```python
from build123d import *

# Parameters (mm, degrees)
F0_W     = 50.8
F0_H     = 50.8
F1_DEPTH = 387.35
F2_SIZE  = 50.79999
F3_W     = 44.45
F3_H     = 44.45
F4_DEPTH = 876.3
F5_R     = 9.525
F7_D     = 12.7
F7_DEPTH = 127
F7_TIP   = 3.8154649308


# Not quite as in the source:
# - a fillet or chamfer is up to 0.001 mm smaller than in the source, because OpenCascade refuses the exact size


with BuildPart() as f1:
    # F0 (on Right) → F1 (new body)
    with BuildSketch(Plane.YZ):
        with Locations((25.4, 25.4)):
            Rectangle(F0_W, F0_H)
    extrude(amount=-F1_DEPTH)

    # F2 (size 50.8 in the source; OpenCascade refuses exactly that, so slightly less here)
    f2_edges = [f1.edges().sort_by_distance(p)[0] for p in [
        (-387.35, 50.8, 25.4),
    ]]
    chamfer(f2_edges, length=F2_SIZE)

    # F3 (on face) → F4 (cut)
    with BuildSketch(Plane.YZ):
        with Locations((25.4, 25.4)):
            Rectangle(F3_W, F3_H)
    extrude(amount=-F4_DEPTH, mode=Mode.SUBTRACT)

    # F5
    f5_edges = [f1.edges().sort_by_distance(p)[0] for p in [
        (-192.087505, 3.175, 3.175),
        (-169.862505, 47.625, 3.175),
        (-169.862505, 47.625, 47.625),
        (-192.087505, 3.175, 47.625),
        (-168.275005, 50.8, 0),
        (-168.275005, 50.8, 50.8),
        (-193.675, 0, 50.8),
        (-193.675, 0, 0),
    ]]
    fillet(f5_edges, radius=F5_R)

    # F7
    with Locations(Plane(origin=(0, 0, 0), x_dir=(1, 0, 0), z_dir=(0, 0, -1))):
        with Locations((-38.1, -31.75), (-63.5, -31.75), (-88.9, -31.75)):
            Hole(F7_D / 2, depth=F7_DEPTH)
            with Locations((0, 0, -(F7_DEPTH + F7_TIP / 2))):  # 118° drill point
                Cone(0, F7_D / 2, F7_TIP, mode=Mode.SUBTRACT)


solid = f1.part
```
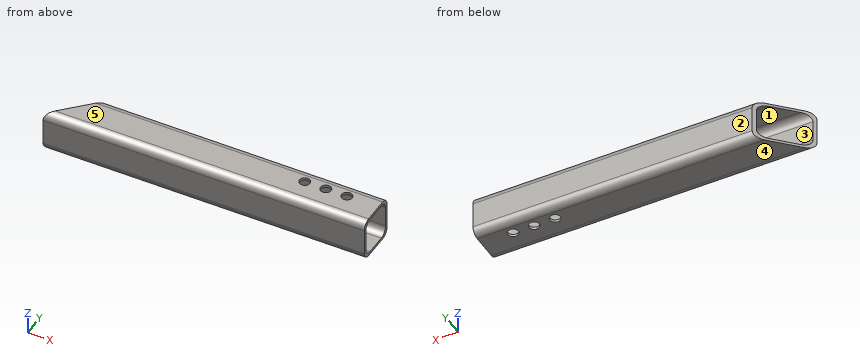
Could you check a few things on this model? Use its own coordinates, in mm. Face numbers are marked on the shaded views. A direction names the side the tool comes from. Round coordinates to 2 decimals unless told otherwise and drop trailing zeros. Write each loop counter-clockwise with the first axis right and the second up, starting at its lowest first coordinate (ties: lowest second). Pieces come first, ordered by that corner, then holes. Notation, with made-up numbers: M -37,70.5 L -17,70.5 A17 cw -17,100.5 Z; hole C -38,73.5 d9. An arc over 180 degrees is marked long. Write each question's results on one line, items separated by ' | '. Start each with the question number.
1. I need wall thicknesses on L1, parallel to Z at x = -70, y = 27 (3 decimals); L2, parallel to X at y = 31.75, z = 50.05. Which ranges of each line are inside material? Lowest first, please. Write a range as from..to.
2. Imagine slicing it at B-B on x = -288. List the corners of the cut face in (y, z) for me (3 decimals).
3. Thinking about a two-plate mould opening in Z: for the marked faces 3, 4 and 5, which applies, +Z half, -Z half, draft (parallel to the pull), parting line (faces both ways), or undercut?
4. Imagine slicing it at C-C on y = 31.75. Count the separate pieces of the cut face and the enclosed holes in it, and give its area (3 significant figures).
5. On a 3-axis mill with a long thin cutter (end or side, diameter ignored), from which of +Z, -Z, +X, -X, +Y, -Y can I reach the whole of each face in a straight line? I mean the marked faces 1 and 2. Say none if no direction works.
Result sheet:
1) L1: z = 0..3.175, 47.625..50.8 | L2: x = -355.6..-95.25, -82.55..-69.85, -57.15..-44.45, -31.75..0
2) outline: M 0,9.525 A9.525 ccw 9.525,0 L 41.275,0 A9.525 ccw 50.8,9.525 L 50.8,41.275 A9.525 ccw 41.275,50.8 L 9.525,50.8 A9.525 ccw 0,41.275 Z; hole M 3.175,12.7 A9.525 ccw 12.7,3.175 L 38.1,3.175 A9.525 ccw 47.625,12.7 L 47.625,38.1 A9.525 ccw 38.1,47.625 L 12.7,47.625 A9.525 ccw 3.175,38.1 Z
3) face 3: undercut | face 4: -Z half | face 5: +Z half
4) separate pieces: 8 | enclosed holes: 0 | area: 2,020 mm^2
5) face 1: +X, -X | face 2: +Z, -Z, +X, -X, +Y
